from build123d import *

# Parameters (mm, degrees)
SKETCH1_R            = 35
BOSS_EXTRUDE1_DEPTH  = 46
BOSS_EXTRUDE2_DEPTH  = 4
EXTRUDE_THIN1_DEPTH  = 16
SKETCH9_R            = 17
CUT_EXTRUDE1_DEPTH   = 44
SKETCH10_R           = 8
CUT_EXTRUDE2_DEPTH   = 10
CHAMFER1_SIZE        = 1
CHAMFER1_SIZE2       = 0.577350269
CHAMFER2_SIZE        = 1
CHAMFER2_SIZE2       = 0.577350269
FILLET1_R            = 1
SHELL2_START         = -49
SHELL2_OUTLINE_R     = 38
SHELL2_OUTLINE_R_2   = 14
SHELL2_DEPTH         = 52
SHELL2_2_DEPTH       = 22
SHELL2_START_2       = -5
SHELL2_3_OUTLINE_R   = 14
SHELL2_3_OUTLINE_R_2 = 5
SHELL2_3_DEPTH       = 8
SHELL2_START_3       = -7
SHELL2_4_DEPTH       = 2
SHELL2_START_4       = -45.0000001
SHELL2_5_OUTLINE_R   = 35
SHELL2_5_OUTLINE_R_2 = 17
SHELL2_5_DEPTH       = 45.0000001
SHELL2_START_5       = -46
SHELL2_6_DEPTH       = 16
SHELL2_START_6       = -4
SHELL2_7_DEPTH       = 4
SHELL2_START_7       = -1.422649831
SHELL2_8_OUTLINE_R   = 17
SHELL2_8_OUTLINE_R_2 = 8
SHELL2_8_DEPTH       = 0.845299462
SKETCH15_R           = 4
CUT_EXTRUDE5_DEPTH   = 2
SKETCH18_R           = 5
CUT_EXTRUDE6_DEPTH   = 1
CIRPATTERN4_COUNT    = 3
SKETCH24_R           = 3
SKETCH24_R_2         = 1
EXTRUDE_THIN2_DEPTH  = 15
CUT_EXTRUDE7_START   = -10
SKETCH24_2_R         = 1
CUT_EXTRUDE7_DEPTH   = 10
SKETCH27_R           = 4
SKETCH27_R_2         = 3
EXTRUDE_THIN3_DEPTH  = 3
SKETCH30_R           = 2
SKETCH30_R_2         = 1
EXTRUDE_THIN5_DEPTH  = 5
SKETCH28_R           = 4
SKETCH28_R_2         = 3
EXTRUDE_THIN6_DEPTH  = 3
SKETCH31_R           = 2
SKETCH31_R_2         = 1
EXTRUDE_THIN7_DEPTH  = 5


with BuildPart() as part:
    # Sketch1 → Boss-Extrude1 (new body)
    with BuildSketch(Plane(origin=(0, 0, 0), x_dir=(1, 0, 0), z_dir=(0, 1, 0))):
        with Locations(Location((0, 0, 0), (0, 0, 270))):
            Circle(SKETCH1_R)
    extrude(amount=-BOSS_EXTRUDE1_DEPTH)

    # Sketch1<3> → Boss-Extrude2 (add)
    with BuildSketch(Plane(origin=(0, 0, 0), x_dir=(1, 0, 0), z_dir=(0, 1, 0))):
        with BuildLine():
            Line((35, -35), (35, 0))
            ThreePointArc((35, 0), (24.748737342, -24.748737342), (0, -35))
            Line((0, -35), (35, -35))
        make_face()
    extrude(amount=-BOSS_EXTRUDE2_DEPTH)

    # Sketch5 → Extrude-Thin1 (add)
    with BuildSketch(Plane.XZ.offset(46)):
        Polygon((0, 35), (-35, 35), (-35, 0), (-25, 0), (-25, 25), (0, 25), align=None)
    extrude(amount=-EXTRUDE_THIN1_DEPTH)

    # Sketch9 → Cut-Extrude1 (cut)
    with BuildSketch(Plane.XZ.offset(46)):
        with Locations(Location((0, 0, 0), (0, 0, 270))):
            Circle(SKETCH9_R)
    extrude(amount=-CUT_EXTRUDE1_DEPTH, mode=Mode.SUBTRACT)

    # Sketch10 → Cut-Extrude2 (cut)
    with BuildSketch(Plane(origin=(0, 0, 0), x_dir=(1, 0, 0), z_dir=(0, 1, 0))):
        with Locations(Location((0, 0, 0), (0, 0, 270))):
            Circle(SKETCH10_R)
    extrude(amount=-CUT_EXTRUDE2_DEPTH, mode=Mode.SUBTRACT)

    # Chamfer1
    chamfer1_edges = [part.edges().sort_by_distance(p)[0] for p in [
        (0, 0, -8),
    ]]
    chamfer1_side = [part.faces().sort_by_distance(p)[0] for p in [
        (-24.048737342, 0, -24.048737342),
    ]]
    chamfer(chamfer1_edges, length=CHAMFER1_SIZE, length2=CHAMFER1_SIZE2, reference=chamfer1_side[0])

    # Chamfer2
    chamfer2_edges = [part.edges().sort_by_distance(p)[0] for p in [
        (0, -2, -8),
    ]]
    chamfer2_side = [part.faces().sort_by_distance(p)[0] for p in [
        (0, -2, 16.519167389),
    ]]
    chamfer(chamfer2_edges, length=CHAMFER2_SIZE, length2=CHAMFER2_SIZE2, reference=chamfer2_side[0])

    # Fillet1
    fillet1_edges = [part.edges().sort_by_distance(p)[0] for p in [
        (0, -46, 17),
    ]]
    fillet(fillet1_edges, radius=FILLET1_R)

    # Shell2: read off the stored shape, not the designer's step
    # Shell2 outline → Shell2 (add)
    with BuildSketch(Plane(origin=(0, 0, 0), x_dir=(1, 0, 0), z_dir=(0, 1, 0)).offset(SHELL2_START)):
        Circle(SHELL2_OUTLINE_R)
        Circle(SHELL2_OUTLINE_R_2, mode=Mode.SUBTRACT)
    extrude(amount=SHELL2_DEPTH)

    # Shell2 2 outline → Shell2 2 (add)
    with BuildSketch(Plane(origin=(0, 0, 0), x_dir=(1, 0, 0), z_dir=(0, 1, 0)).offset(SHELL2_START)):
        with BuildLine():
            ThreePointArc((0, -38), (-26.870057685, -26.870057685), (-38, 0))
            Line((-38, 0), (-38, -38))
            Line((-38, -38), (0, -38))
        make_face()
    extrude(amount=SHELL2_2_DEPTH)

    # Shell2 3 outline → Shell2 3 (add)
    # profile 1 of 2: a face of its own
    with BuildSketch(Plane(origin=(0, 0, 0), x_dir=(1, 0, 0), z_dir=(0, 1, 0)).offset(SHELL2_START_2)):
        with BuildLine():
            Line((38, -38), (38, 0))
            ThreePointArc((38, 0), (26.870057685, -26.870057685), (0, -38))
            Line((0, -38), (38, -38))
        make_face()
    # profile 2 of 2: a face of its own
    with BuildSketch(Plane(origin=(0, 0, 0), x_dir=(1, 0, 0), z_dir=(0, 1, 0)).offset(SHELL2_START_2)):
        Circle(SHELL2_3_OUTLINE_R)
        Circle(SHELL2_3_OUTLINE_R_2, mode=Mode.SUBTRACT)
    extrude(amount=SHELL2_3_DEPTH)

    # Shell2 4 outline → Shell2 4 (add)
    with BuildSketch(Plane(origin=(0, 0, 0), x_dir=(1, 0, 0), z_dir=(0, 1, 0)).offset(SHELL2_START_3)):
        with BuildLine():
            Line((38, -38), (38, 0))
            ThreePointArc((38, 0), (26.870057685, -26.870057685), (0, -38))
            Line((0, -38), (38, -38))
        make_face()
    extrude(amount=SHELL2_4_DEPTH)

    # Shell2 5 outline → Shell2 5 (cut)
    with BuildSketch(Plane(origin=(0, 0, 0), x_dir=(1, 0, 0), z_dir=(0, 1, 0)).offset(SHELL2_START_4)):
        Circle(SHELL2_5_OUTLINE_R)
        Circle(SHELL2_5_OUTLINE_R_2, mode=Mode.SUBTRACT)
    extrude(amount=SHELL2_5_DEPTH, mode=Mode.SUBTRACT)

    # Shell2 6 outline → Shell2 6 (cut)
    with BuildSketch(Plane(origin=(0, 0, 0), x_dir=(1, 0, 0), z_dir=(0, 1, 0)).offset(SHELL2_START_5)):
        with BuildLine():
            ThreePointArc((-25, -24.494897428), (-32.403703492, -13.228756555), (-35, 0))
            Line((-35, 0), (-35, -35))
            Line((-35, -35), (0, -35))
            ThreePointArc((0, -35), (-13.228756555, -32.403703492), (-24.494897428, -25))
            Line((-24.494897428, -25), (-25, -25))
            Line((-25, -25), (-25, -24.494897428))
        make_face()
    extrude(amount=SHELL2_6_DEPTH, mode=Mode.SUBTRACT)

    # Shell2 7 outline → Shell2 7 (cut)
    with BuildSketch(Plane(origin=(0, 0, 0), x_dir=(1, 0, 0), z_dir=(0, 1, 0)).offset(SHELL2_START_6)):
        with BuildLine():
            Line((35, -35), (35, 0))
            ThreePointArc((35, 0), (24.748737342, -24.748737342), (0, -35))
            Line((0, -35), (35, -35))
        make_face()
    extrude(amount=SHELL2_7_DEPTH, mode=Mode.SUBTRACT)

    # Shell2 8 outline → Shell2 8 (cut)
    with BuildSketch(Plane(origin=(0, 0, 0), x_dir=(1, 0, 0), z_dir=(0, 1, 0)).offset(SHELL2_START_7)):
        Circle(SHELL2_8_OUTLINE_R)
        Circle(SHELL2_8_OUTLINE_R_2, mode=Mode.SUBTRACT)
    extrude(amount=SHELL2_8_DEPTH, mode=Mode.SUBTRACT)

    # Shell2 9 outline → Shell2 9 (revolve, cut)
    with BuildSketch(Plane.XY):
        Polygon((5, 3), (5, 1.154700538), (8.196152423, 3), align=None)
        Polygon((17, -0.577350369), (17, 0), (9, 0), (8, -0.577350319), align=None)
        Polygon((8, -1.422649781), (9, -2), (17, -2), (17, -1.422649831), align=None)
        Polygon((8.196152423, -5), (5, -3.154700538), (5, -5), align=None)
        with BuildLine():
            Line((14, -45), (14, -49))
            Line((14, -49), (18, -49))
            ThreePointArc((18, -49), (15.171572875, -47.828427125), (14, -45))
        make_face()
        with BuildLine():
            ThreePointArc((17, -45), (17.292893219, -45.707106781), (18, -46))
            Line((18, -46), (35, -46))
            Line((35, -46), (35, -45.0000001))
            Line((35, -45.0000001), (17, -45))
        make_face()
    revolve(axis=Axis((0, 0, 0), (0, 1, 0)), mode=Mode.SUBTRACT)

    # Sketch15 → Cut-Extrude5 (cut)
    with BuildSketch(Plane.XZ.offset(49)):
        with Locations(Location((0, 24, 0), (0, 0, 270))):
            Circle(SKETCH15_R)
    cut_extrude5 = extrude(amount=-CUT_EXTRUDE5_DEPTH, mode=Mode.SUBTRACT)

    # Sketch18 → Cut-Extrude6 (cut)
    with BuildSketch(Plane.XZ.offset(49)):
        with Locations(Location((0, 24, 0), (0, 0, 270))):
            Circle(SKETCH18_R)
    cut_extrude6 = extrude(amount=-CUT_EXTRUDE6_DEPTH, mode=Mode.SUBTRACT)

    # CirPattern4: Cut-Extrude5, Cut-Extrude6 ×3 about axis
    cirpattern4_axis = Axis((0, 0, 0), (0, 1, 0))
    add([cut_extrude5.rotate(cirpattern4_axis, i * 360 / CIRPATTERN4_COUNT) for i in range(1, CIRPATTERN4_COUNT)], mode=Mode.SUBTRACT)
    add([cut_extrude6.rotate(cirpattern4_axis, i * 360 / CIRPATTERN4_COUNT) for i in range(1, CIRPATTERN4_COUNT)], mode=Mode.SUBTRACT)

    # Sketch24 → Extrude-Thin2 (add)
    # profile 1 of 2: a face of its own
    with BuildSketch(Plane.XY.offset(38)):
        with Locations((-19, -39)):
            Circle(SKETCH24_R)
        with Locations((-19, -39)):
            Circle(SKETCH24_R_2, mode=Mode.SUBTRACT)
    # profile 2 of 2: a face of its own
    with BuildSketch(Plane.XY.offset(38)):
        with Locations((19, -2)):
            Circle(SKETCH24_R)
        with Locations((19, -2)):
            Circle(SKETCH24_R_2, mode=Mode.SUBTRACT)
    extrude(amount=EXTRUDE_THIN2_DEPTH)

    # Sketch24<2> → Cut-Extrude7 (cut)
    with BuildSketch(Plane.XY.offset(38).offset(CUT_EXTRUDE7_START)):
        with Locations((-19, -39)):
            Circle(SKETCH24_2_R)
        with Locations(Location((19, -2, 0), (0, 0, 180))):
            Circle(SKETCH24_2_R)
    extrude(amount=CUT_EXTRUDE7_DEPTH, mode=Mode.SUBTRACT)

    # Sketch27 → Extrude-Thin3 (add)
    with BuildSketch(Plane.XY.offset(50)):
        with Locations((19, -2)):
            Circle(SKETCH27_R)
        with Locations((19, -2)):
            Circle(SKETCH27_R_2, mode=Mode.SUBTRACT)
    extrude(amount=EXTRUDE_THIN3_DEPTH)

    # Sketch30 → Extrude-Thin5 (add)
    with BuildSketch(Plane.XY.offset(50)):
        with Locations((19, -2)):
            Circle(SKETCH30_R)
        with Locations((19, -2)):
            Circle(SKETCH30_R_2, mode=Mode.SUBTRACT)
    extrude(amount=EXTRUDE_THIN5_DEPTH)

    # Sketch28 → Extrude-Thin6 (add)
    with BuildSketch(Plane.XY.offset(50)):
        with Locations((-19, -39)):
            Circle(SKETCH28_R)
        with Locations((-19, -39)):
            Circle(SKETCH28_R_2, mode=Mode.SUBTRACT)
    extrude(amount=EXTRUDE_THIN6_DEPTH)

    # Sketch31 → Extrude-Thin7 (add)
    with BuildSketch(Plane.XY.offset(50)):
        with Locations((-19, -39)):
            Circle(SKETCH31_R)
        with Locations((-19, -39)):
            Circle(SKETCH31_R_2, mode=Mode.SUBTRACT)
    extrude(amount=EXTRUDE_THIN7_DEPTH)


solid = part.part
Design review of the part built by this model. Coordinates are the model's own, in mm. A direction names the side the tool comes from. Round coordinates to 2 decimals unless told otherwise and drop trailing zeros. Write each loop counter-clockwise with the first axis right and the second up, starting at its lowest first coordinate (ties: lowest second). Pieces come first, ordered by that corner, then holes. Notation, with made-up numbers: (20.25, 0) -> (54.25, 0) arc R26 ccw to (54.25, 28) -> close; hole circle Ø2 at (74, 65.5). An arc over 180 degrees is marked (long way). One line per question, with ' | ' between items.
(1) Insertion check: P1, Ø10, axis at x = -23.5, y = -25.5, coming from the -Z side; P2, Ø1.5, axis at x = -9.5, y = -8, coming from the -Z side; P3, Ø5, axis at y = -35, z = 11.5, coming from the +X side. Each pin has a flat end and moves straight along its axis. Give the tip position at first contact, or say it passes through.
Result sheet:
P1: z = -33.19 | P2: z = -36.98 | P3: x = 36.92
(2) Take a section at B-B, the plane x = 30.5. State the section outline as (y, z) points.
Result sheet:
outline: (-49, -22.67) -> (3, -22.67) -> (3, 38) -> (-7, 38) -> (-7, 22.67) -> (-49, 22.67) -> close; hole (-46, -17.17) -> (0, -17.17) -> (0, 35) -> (-4, 35) -> (-4, 17.17) -> (-46, 17.17) -> close
(3) Take a section at C-C, the plane y = -23. State the section outline as (x, z) points.
Result sheet:
outline: circle Ø76 at (0, 0); circle Ø34 at (0, 0); hole circle Ø70 at (0, 0); hole circle Ø28 at (0, 0)
(4) Draft analysis for pull direction Y (two halves, no side actions). For faces 1 (the conical face through (-1.127, 1.27, 5.076)), 2 (the cylindrical face through (23.488, -47.507, -9.052)), 3 (the flat face through (-7, -2, 7)), state which applies: released by +Y, released by -Y, zero draft, split by the parting line, or undercut.
Result sheet:
face 1: released by +Y | face 2: zero draft | face 3: undercut
(5) Machinability: for faces 4 (the cylindrical face through (-1.08, -1.03, 4.88)), 5 (the flat face through (-38, -38, 19)), 6 (the flat face through (-18, -37, 53)), 7 (the cylindrical face through (-2.4, -47.5, 27.2)), 8 (the flat face through (-28, -30, 26)), which of the approach directions +Z, -Z, +X, -X, +Y, -Y give a long, thin tool a straight path to every point of the face, cutting with its end or side? Answer none if there is none.
Result sheet:
face 4: +Y, -Y | face 5: +Z, -Z, -X, +Y, -Y | face 6: +Z | face 7: -Y | face 8: none
(6) Take a section at A-A, the plane y = -31.5. State the section outline as (x, z) points, and give its area (3 significant figures).
Result sheet:
outline: (-38, 0) arc R38 ccw (long way) to (0, 38) -> (-38, 38) -> close; (-25, 24.49) arc R35 cw to (-24.49, 25) -> (-25, 25) -> close; circle Ø34 at (0, 0); hole (-35, 0) arc R35 ccw (long way) to (0, 35) -> (-35, 35) -> close; hole circle Ø28 at (0, 0) | area: 1,030 mm2
(7) Wall thickness on line 1 (Y direction, x = 19, z = 54.5); line 2 (X direction, y = -47.6, z = -12); line 3 (X direction, y = -9, z = -11.5): over which ranges is each line inside the solid? List them lowest first. Write a range as [from, to].
Result sheet:
line 1: [-4, -3], [-1, 0] | line 2: [-36.06, -24.78], [-16.78, -8.93], [8.93, 16.78], [24.78, 36.06] | line 3: [-36.22, -33.06], [-12.52, -7.98], [7.98, 12.52], [33.06, 36.22]
(8) Take a section at D-D, the plane z = -27. State the section outline as (x, y) points.
Result sheet:
outline: (-26.74, -49) -> (26.74, -49) -> (26.74, 3) -> (-26.74, 3) -> close; hole (-22.27, -46) -> (22.27, -46) -> (22.27, 0) -> (-22.27, 0) -> close
